Autodesk Inventor part; units mm, degrees
ref_plane "Pracovní rovina1" through (1.5, 0, 0) normal (1, 0, 0) x (0, 0, -1)
ref_plane "Pracovní rovina2" through (-1.5, 0, 0) normal (-1, 0, 0) x (0, 0, 1)
ref_plane "YZ Plane" through (0, 0, 0) normal (1, 0, 0) x (0, 1, 0)
sketch "Náčrt1" plane through (0, 0, 0) normal (1, 0, 0) x (0, 1, 0)
  line L0 (19, 6.35) -> (31.312, 6.35)
  line L1 (31.312, -6.35) -> (19, -6.35)
  line L2 (19, -6.35) -> (19, 6.35)
  line L3 (24.7725, 20.1763) -> (16.7938, 12.1976)
  line L4 (16.7938, 12.1976) -> (12.1976, 16.7938)
  line L5 (12.1976, 16.7938) -> (20.1763, 24.7725)
  line L6 (0, 0) -> (14.4957, 14.4957)
  line L7 (6.35, 19) -> (-6.35, 19)
  line L8 (6.35, 31.312) -> (6.35, 19)
  line L9 (-6.35, 19) -> (-6.35, 31.312)
  line L10 (-20.1763, 24.7725) -> (-12.1976, 16.7938)
  line L11 (-12.1976, 16.7938) -> (-16.7938, 12.1976)
  line L12 (-16.7938, 12.1976) -> (-24.7725, 20.1763)
  line L13 (-19, 6.35) -> (-19, -6.35)
  line L14 (-31.312, 6.35) -> (-19, 6.35)
  line L15 (-19, -6.35) -> (-31.312, -6.35)
  line L16 (-24.7725, -20.1763) -> (-16.7938, -12.1976)
  line L17 (-16.7938, -12.1976) -> (-12.1976, -16.7938)
  line L18 (-12.1976, -16.7938) -> (-20.1763, -24.7725)
  line L19 (-6.35, -19) -> (6.35, -19)
  line L20 (-6.35, -31.312) -> (-6.35, -19)
  line L21 (6.35, -19) -> (6.35, -31.312)
  line L22 (20.1763, -24.7725) -> (12.1976, -16.7938)
  line L23 (12.1976, -16.7938) -> (16.7938, -12.1976)
  line L24 (16.7938, -12.1976) -> (24.7725, -20.1763)
  arc A0 (24.7725, -20.1763) -> (31.312, -6.35) centre (0, 0) ccw
  arc A1 (6.35, -31.312) -> (20.1763, -24.7725) centre (0, 0) ccw
  arc A2 (-20.1763, -24.7725) -> (-6.35, -31.312) centre (0, 0) ccw
  arc A3 (-31.312, -6.35) -> (-24.7725, -20.1763) centre (0, 0) ccw
  arc A4 (-24.7725, 20.1763) -> (-31.312, 6.35) centre (0, 0) ccw
  arc A5 (-6.35, 31.312) -> (-20.1763, 24.7725) centre (0, 0) ccw
  arc A6 (31.312, 6.35) -> (24.7725, 20.1763) centre (0, 0) ccw
  arc A7 (20.1763, 24.7725) -> (6.35, 31.312) centre (0, 0) ccw
  line L25 (16.187, 20.7832) -> (20.7832, 16.187)
  line L26 (14.9495, 23.4348) -> (13.5353, 22.0206)
  line L27 (13.5353, 22.0206) -> (22.0206, 13.5353)
  line L28 (22.0206, 13.5353) -> (23.4348, 14.9495)
  line L29 (23.4348, 14.9495) -> (14.9495, 23.4348)
  line L30 (-13.5353, 22.0206) -> (-14.9495, 23.4348)
  line L31 (-22.0206, 13.5353) -> (-13.5353, 22.0206)
  line L32 (-14.9495, 23.4348) -> (-23.4348, 14.9495)
  line L33 (-23.4348, 14.9495) -> (-22.0206, 13.5353)
  line L34 (-22.0206, -13.5353) -> (-23.4348, -14.9495)
  line L35 (-13.5353, -22.0206) -> (-22.0206, -13.5353)
  line L36 (-23.4348, -14.9495) -> (-14.9495, -23.4348)
  line L37 (-14.9495, -23.4348) -> (-13.5353, -22.0206)
  line L38 (13.5353, -22.0206) -> (14.9495, -23.4348)
  line L39 (22.0206, -13.5353) -> (13.5353, -22.0206)
  line L40 (14.9495, -23.4348) -> (23.4348, -14.9495)
  line L41 (23.4348, -14.9495) -> (22.0206, -13.5353)
  point P0 (-14.4957, 14.4957)
  point P1 (-14.4957, -14.4957)
  point P2 (14.4957, -14.4957)
  dimension "d1" = 6.35
  dimension "d2" = 6.35
  dimension "d4" = 6.5
  dimension "d5" = 3.25
  dimension "d6" = 20.5
  dimension "d7" = 45
  dimension "d10" = 360
  dimension "d12" = 2
  dimension "d13" = 12
  dimension "d14" = 1
  dimension "d15" = 2.75
  dimension "d18" = 360
extrude "Vysunutí1" add sketch "Náčrt1" along normal mid plane 3 contours L2 L1 A0 L24 L40 L41 L39 L23 L22 L38 A1 L21 L19 L20 A2 L18 L36 L37 L35 L17 L16 L34 A3 L15 L13 L14 A4 L12 L32 L33 L31 L11 L10 L30 A5 L9 L7 L8 A7 L5 L29 L26 L27 L4 L3 L28 A6 L0 | L29 L28 L27 L3 | L5 L27 L26 L29 | L24 L39 L41 L40 | L40 L38 L39 L22 | L32 L30 L31 L10 | L12 L31 L33 L32 | L18 L35 L37 L36 | L36 L34 L35 L16
ref_plane "Pracovní rovina1" through (1.5, 0, 0) normal (1, 0, 0) x (0, 0, -1)
sketch "Náčrt3" plane through (1.5, 0, 0) normal (1, 0, 0) x (0, 0, -1)
  line L0 (-11.5, 7) -> (-11.5, -7)
  line L1 (11.5, -7) -> (11.5, 7)
  arc A0 (5, 7) -> (-5, 7) centre (0, 7) ccw
  arc A1 (-5, -7) -> (5, -7) centre (0, -7) ccw
  line L2 (-11.5, -7) -> (-5, -7)
  line L3 (5, -7) -> (11.5, -7)
  line L4 (11.5, 7) -> (5, 7)
  line L5 (-5, 7) -> (-11.5, 7)
  point P0 (0, 0)
  dimension "d34" = 23
  dimension "d35" = 14
  dimension "d37" = 11.5
  dimension "d38" = 10
  dimension "d39" = 10
extrude "Vysunutí3" cut sketch "Náčrt3" against normal blind 4
ref_plane "Pracovní rovina2" through (-1.5, 0, 0) normal (-1, 0, 0) x (0, 0, 1)
sketch "Náčrt6" plane through (-1.5, 0, 0) normal (1, 0, 0) x (0, 0, -1)
  circle A0 centre (10, 23) radius 1.55
  circle A1 centre (-10, 23) radius 1.55
  circle A2 centre (-23, 10) radius 1.55
  circle A3 centre (-23, -10) radius 1.55
  circle A4 centre (-10, -23) radius 1.55
  circle A5 centre (10, -23) radius 1.55
  circle A6 centre (23, -10) radius 1.55
  circle A7 centre (23, 10) radius 1.55
  point P0 (0, 0)
  dimension "d52" = 3.1
  dimension "d53" = 3.1
  dimension "d54" = 23
  dimension "d55" = 23
  dimension "d56" = 10
  dimension "d57" = 10
  dimension "d60" = 360
sketch "Sketch7" plane through (-1.5, 16.7938, 12.1976) normal (0, -0.7071, 0.7071) x (1, 0, 0)
  circle A0 centre (2.9795, 2.2836) radius 1
  line L0 (0, 11.2836) -> (3, 11.2836)
  point P0 (1.5, -20.5)
  dimension "d64" = 2
  dimension "d65" = 9
extrude "Extrusion6" cut sketch "Sketch7" against normal blind 3 and the other way blind 9
pattern_circular "Circular Pattern1" count 4 over 360 about axis through (0, 0, 0) along (1, 0, 0) of "Extrusion6"
hole "Hole3" at (-1.5, 10, 23) at (-1.5, 23, 10) at (-1.5, -10, 23) at (-1.5, -23, 10) at (-1.5, -23, -10) at (-1.5, 23, -10) at (-1.5, 10, -23) at (-1.5, -10, -23) direction (1, 0, 0) diameter 3.1 end through all countersink diameter 6 countersink angle 90
equation "\"d5\" = 0.5 * d4"
equation "\"d14\" = 0.5 * d12"
equation "\"d15\" = -0.5 * d4 + 0.5 * d13"
equation "\"d39\" = d38"
equation "\"d36\" = 0.5 * d35"
properties part number "deska"
Geometry: final body of the model. Coordinates: model frame, mm. A direction names the side the tool comes from. Coordinates: 2 decimals unless noted, no trailing zeros. Loops run counter-clockwise (first coordinate to the right, second up) from the corner with the lowest first, then second, coordinate; pieces in that order, holes last. Notation, with made-up numbers: (-27.75, 47.25) -> (14.25, 47.25) arc R26 cw to (14.25, 75.25) -> close; hole circle Ø3 at (77.25, 87.5). An arc over 180 degrees is marked (long way). Use a Markdown table: item, result. Add a question column.
(1) Line query: line 1 along Z through (x, y) = (1.15, -10); line 2 along Y through (x, z) = (1.2, -23); line 3 along Z through (x, y) = (-1.4, -2.5). Output: solid intervals per line, ascending.
(2) Section query D-D, the plane x = -1. State how many separate pieces and enclosed holes the cut face has, plus the area to 3 significant figures.
(3) Section query B-B, the plane y = -1.5. Return loops of the section in (x, z).
(4) Section query A-A, the plane z = 0. Return loops of the section in (x, y).
(5) Mould query, pull axis Y, two halves, no side actions, for faces 1 (the flat face through (1.5, -7.4, 7.4)), 2 (the cylindrical face through (-0.021, -13.758, 28.835)), 3 (the flat face through (0, 6.35, 25)), 4 (the flat face through (0, 7, -8)). Classes: pulls with the +Y half, pulls with the -Y half, needs draft (parallel to the pull), parting line crosses it, or undercut.
(6) Pin query (flat end, axial travel): pin 1 Ø1.5 at (x, z) = (1, 17) entering from -Y; pin 2 Ø3 at (y, z) = (10, -23) entering from -X; pin 3 Ø1.5 at (x, z) = (0.5, -9) entering from -Y; pin 4 Ø0.9 at (x, z) = (-0.5, 7.5) entering from -Y. Return the tip coordinate at first contact, or that it passes through.
(7) Section query C-C, the plane z = -23. Return loops of the section in (x, y), plus the area to 3 significant figures.
(8) Access query for faces 5 (the flat face through (1.096, -20.188, 12.053)), 6 (the flat face through (-0.02, 14.53, 14.46)), 7 (the flat face through (0, 25, 6.35)). Directions: +Z, -Z, +X, -X, +Y, -Y. A direction counts if a zero-diameter tool reaches every point of the face in a straight line with its end or side. Return the directions, or none.
Answer:
| question | item | result |
|---|---|---|
| 1 | line 1 | z = -30.34 to -24.55, -21.45 to -4, 4 to 21.45, 24.55 to 30.34 |
| 1 | line 2 | y = -18.4 to -11.55, -8.45 to -6.35, 6.35 to 8.45, 11.55 to 18.4 |
| 1 | line 3 | z = -19 to -11.5, 11.5 to 19 |
| 2 | separate pieces | 1 |
| 2 | enclosed holes | 9 |
| 2 | area | 1,710 mm^2 |
| 3 | outline | (-1.5, -19) -> (1.5, -19) -> (1.5, -11.5) -> (-1.5, -11.5) -> close; (-1.5, 11.5) -> (1.5, 11.5) -> (1.5, 19) -> (-1.5, 19) -> close |
| 4 | outline | (-1.5, -19) -> (1.5, -19) -> (1.5, -12) -> (-1.5, -12) -> close; (-1.5, 12) -> (1.5, 12) -> (1.5, 19) -> (-1.5, 19) -> close |
| 5 | face 1 | needs draft |
| 5 | face 2 | pulls with the -Y half |
| 5 | face 3 | undercut |
| 5 | face 4 | undercut |
| 6 | pin 1 | stops at y = -27.51 |
| 6 | pin 2 | passes through |
| 6 | pin 3 | stops at y = -30.87 |
| 6 | pin 4 | stops at y = -31.16 |
| 7 | outline | (-1.5, -18.4) -> (1.5, -18.4) -> (1.5, -11.55) -> (-0.05, -11.55) -> (-1.5, -13) -> close; (-1.5, -7) -> (-0.05, -8.45) -> (1.5, -8.45) -> (1.5, -6.35) -> (-1.5, -6.35) -> close; (-1.5, 6.35) -> (1.5, 6.35) -> (1.5, 8.45) -> (-0.05, 8.45) -> (-1.5, 7) -> close; (-1.5, 13) -> (-0.05, 11.55) -> (1.5, 11.55) -> (1.5, 18.4) -> (-1.5, 18.4) -> close |
| 7 | area | 49.5 mm^2 |
| 8 | face 5 | +X |
| 8 | face 6 | +X, -X |
| 8 | face 7 | +X, -X, +Y |
